Design review of the part built by this model. Coordinates are the model's own, in mm. A direction names the side the tool comes from. Coordinates: 2 decimals unless noted, no trailing zeros. Write each loop counter-clockwise with the first axis right and the second up, starting at its lowest first coordinate (ties: lowest second). Pieces come first, ordered by that corner, then holes. Notation, with made-up numbers: (-26.75, -36) -> (-15.75, -36) arc R20 ccw to (-15.75, -4) -> close; hole circle Ø1 at (79.5, 25.5). An arc over 180 degrees is marked (long way). One line per question, with ' | ' between items. Start each with the question number.
Q1. For P1, Ø1.6, axis at x = -1.5, z = -0.5, coming from the -Y side; P2, Ø1, axis at y = 1, z = 1.5, coming from the -X side; P3, Ø0.5, axis at y = 1, z = 0, coming from the +X side; P4, Ø2, axis at x = 0, z = 0, coming from the +Y side, all flat-tipped, find the tip position at first contact; note any pin that passes through.
Q2. Add section D-D on y = -2.75. State the section outline as (x, z) points (3 decimals), and give its area (3 significant figures).
Q3. Wall thickness on probe 1 along Y at (x, z) = (-2.1, 1.3); probe 2 along Z at (x, y) = (0.05, -4); probe 3 along X at (y, z) = (3.5, 0) (3 decimals): over which ranges is each line inside the solid? List them lowest first.
Q4. Add section B-B on y = 0.5. State the section outline as (x, z) points (3 decimals).
Q5. Add section C-C on y = 2. State the section outline as (x, z) points (3 decimals), and give its area (3 significant figures).
Q6. Draft analysis for pull direction Y (two halves, no side actions). For faces 4 (the flat face through (2, 1.2, -1)), 5 (the cylindrical face through (2, 0.59, 1.96)), 6 (the flat face through (0, 1.2, 0)), state which applies: pulls with the +Y half, pulls with the -Y half, needs draft (parallel to the pull), parting line crosses it, or undercut.
Q7. For faces 1 (the flat face through (2.4, 1, 0)), 2 (the cylindrical face through (2.03, 0.59, -1.93)), 3 (the flat face through (0, 0, 0)), list the 3-axis set-ups (+Z, -Z, +X, -X, +Y, -Y) from which the entire face can be reached by the end or side of a thin tool; tool diameter is ignored.
from build123d import *

# Parameters (mm, degrees)
SKETCH1_R           = 2.8
BOSS_EXTRUDE1_DEPTH = 1.2
SKETCH2_R           = 2.065
BOSS_EXTRUDE2_DEPTH = 0.13
SKETCH3_R           = 1.785
BOSS_EXTRUDE3_DEPTH = 2.22
SKETCH4_R           = 0.615
CUT_EXTRUDE1_DEPTH  = 1
SKETCH5_R           = 0.4
BOSS_EXTRUDE4_DEPTH = 0.05
SKETCH6_W           = 0.4
SKETCH6_H           = 1
CUT_EXTRUDE2_DEPTH  = 6.31812937
SKETCH7_R           = 0.6
BOSS_EXTRUDE5_DEPTH = 0.4
SKETCH8_R           = 0.225
BOSS_EXTRUDE6_DEPTH = 6
FILLET1_R           = 0.1
SKETCH9_R           = 1.655
CUT_EXTRUDE3_DEPTH  = 2.22


with BuildPart() as part:
    # Sketch1 → Boss-Extrude1 (new body)
    with BuildSketch(Plane(origin=(0, 0, 0), x_dir=(1, 0, 0), z_dir=(0, 1, 0))):
        with Locations(Location((0, 0, 0), (0, 0, 270))):
            Circle(SKETCH1_R)
    extrude(amount=BOSS_EXTRUDE1_DEPTH)

    # Sketch2 → Boss-Extrude2 (add)
    with BuildSketch(Plane(origin=(0, 1.2, 0), x_dir=(1, 0, 0), z_dir=(0, 1, 0))):
        with Locations(Location((0, 0, 0), (0, 0, 270))):
            Circle(SKETCH2_R)
    extrude(amount=BOSS_EXTRUDE2_DEPTH)

    # Sketch3 → Boss-Extrude3 (add)
    with BuildSketch(Plane(origin=(0, 1.33, 0), x_dir=(1, 0, 0), z_dir=(0, 1, 0))):
        with Locations(Location((0, 0, 0), (0, 0, 270))):
            Circle(SKETCH3_R)
    extrude(amount=BOSS_EXTRUDE3_DEPTH)

    # Sketch4 → Cut-Extrude1 (cut)
    with BuildSketch(Plane(origin=(0, 3.55, 0), x_dir=(1, 0, 0), z_dir=(0, 1, 0))):
        with Locations(Location((0, 0, 0), (0, 0, 270))):
            Circle(SKETCH4_R)
    extrude(amount=-CUT_EXTRUDE1_DEPTH, mode=Mode.SUBTRACT)

    # Sketch5 → Boss-Extrude4 (add)
    with BuildSketch(Plane.XZ):
        with Locations(Location((0, 1, 0), (0, 0, 90))):
            Circle(SKETCH5_R)
        with Locations(Location((0, -1, 0), (0, 0, 90))):
            Circle(SKETCH5_R)
    extrude(amount=BOSS_EXTRUDE4_DEPTH)

    # Sketch6 → Cut-Extrude2 (cut, through all)
    with BuildSketch(Plane.XZ):
        Polygon((0, 2.15), (0.65, 2.8), (-0.65, 2.8), align=None)
        with Locations((2.6, 0)):
            Rectangle(SKETCH6_W, SKETCH6_H)
        Polygon((0, -2.15), (-0.65, -2.8), (0.65, -2.8), align=None)
    extrude(amount=-CUT_EXTRUDE2_DEPTH, mode=Mode.SUBTRACT)

    # Sketch7 → Boss-Extrude5 (add)
    with BuildSketch(Plane.XZ):
        with Locations(Location((1, 0, 0), (0, 0, 90))):
            Circle(SKETCH7_R)
    extrude(amount=BOSS_EXTRUDE5_DEPTH)

    # Sketch8 → Boss-Extrude6 (add)
    with BuildSketch(Plane.XZ.offset(0.05)):
        with Locations(Location((0, 1, 0), (0, 0, 270))):
            Circle(SKETCH8_R)
        with Locations(Location((0, -1, 0), (0, 0, 270))):
            Circle(SKETCH8_R)
        with Locations(Location((1, 0, 0), (0, 0, 270))):
            Circle(SKETCH8_R)
    extrude(amount=BOSS_EXTRUDE6_DEPTH)

    # Fillet1
    fillet1_edges = [part.edges().sort_by_distance(p)[0] for p in [
        (0, 1.33, -1.785),
        (0, 3.55, -1.785),
    ]]
    fillet(fillet1_edges, radius=FILLET1_R)

    # Sketch9 → Cut-Extrude3 (cut)
    with BuildSketch(Plane(origin=(0, 1.2, 0), x_dir=(1, 0, 0), z_dir=(0, 1, 0))):
        with Locations(Location((0, 0, 0), (0, 0, 270))):
            Circle(SKETCH9_R)
    extrude(amount=CUT_EXTRUDE3_DEPTH, mode=Mode.SUBTRACT)


solid = part.part
Output values:
1) P1: stops at y = 0 | P2: stops at x = -2.62 | P3: stops at x = 2.4 | P4: stops at y = 3.55
2) outline: circle Ø0.45 at (0, -1); circle Ø0.45 at (0, 1); circle Ø0.45 at (1, 0) | area: 0.477 mm2
3) probe 1: y = 0 to 1.2 | probe 2: z = -1.22 to -0.78, 0.78 to 1.22 | probe 3: x = -1.772 to -0.615, 0.615 to 1.772
4) outline: (-0.588, -2.738) -> (0, -2.15) -> (0.588, -2.738) arc R2.8 ccw to (2.755, -0.5) -> (2.4, -0.5) -> (2.4, 0.5) -> (2.755, 0.5) arc R2.8 ccw to (0.588, 2.738) -> (0, 2.15) -> (-0.588, 2.738) arc R2.8 ccw to start
5) outline: circle Ø3.57 at (0, 0); hole circle Ø3.31 at (0, 0) | area: 1.40 mm2
6) face 4: pulls with the +Y half | face 5: needs draft | face 6: undercut
7) face 1: +X, +Y, -Y | face 2: -Z, +X, +Y, -Y | face 3: -Y
